Study the drawing (mm; zero at the part's minimum x, y, z) and answer. A direction names the side the tool comes from. Coordinates: 2 decimals unless noted, no trailing zeros. Write each loop counter-clockwise with the first axis right and the second up, starting at its lowest first coordinate (ties: lowest second). Pieces come first, ordered by that corner, then holes. Notation, with made-up numbers: (4.25, 42) -> (52.25, 42) arc R10 ccw to (52.25, 52) -> close; hole circle Ø9 at (-30, 33.25). An arc over 180 degrees is marked (long way). Write item = value, one per line. Start each with the question number.
1) Section B-B (x = 20) is taken. Determine the outline of the cut face in (y, z), plus the area to 3 significant figures.
2) Section C-C (y = 12) is taken. Determine the outline of the cut face in (x, z).
3) For a pull along Y with two mould halves and no side action, classify the marked faces 1, 2 and 3 as released by +Y, released by -Y, zero draft, split by the parting line, or undercut.
4) Section A-A (z = 17.25) is taken. Determine the outline of the cut face in (x, y), plus the area to 3 significant figures.
5) Section D-D (z = 3.75) is taken. Determine the outline of the cut face in (x, y).
6) Flat-ended cylindrical pins translate along their axes: pin 1 Ø6 at (y, z) = (35, 20.5) entering from -X; pin 2 Ø7.5 at (x, y) = (20, 19.5) entering from +Z; pin 3 Ø4 at (x, z) = (29, 16.5) entering from -Y (3 decimals). Find the tip coordinate at first contact, or state that the pin passes through.
7) Find the intervals of material crossed by line 1 along Z through (x, y) = (16, 12.5); line 2 along Y through (x, z) = (20, 14.5); line 3 along X through (y, z) = (23.5, 10.5), in increasing order. Write a range as from..to.
8) A tool of negligible diameter and unlimited length cuts with its end or side. For the marked faces 4 and 5, from which of +Z, -Z, +X, -X, +Y, -Y can it reach the whole face along a straight path? Write none if from no direction.
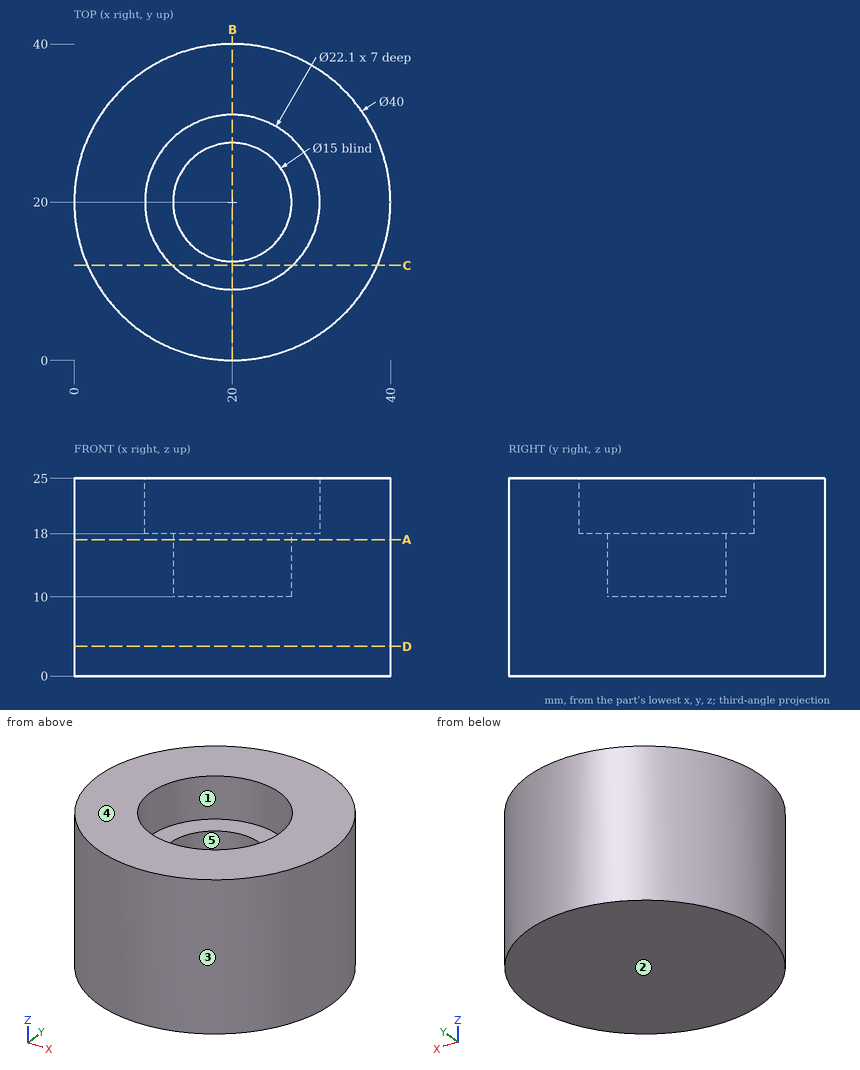
Answer key:
q1.outline = (0, 0) -> (40, 0) -> (40, 25) -> (31.05, 25) -> (31.05, 18) -> (27.5, 18) -> (27.5, 10) -> (12.5, 10) -> (12.5, 18) -> (8.95, 18) -> (8.95, 25) -> (0, 25) -> close
q1.area = 725 mm^2
q2.outline = (1.67, 0) -> (38.33, 0) -> (38.33, 25) -> (27.62, 25) -> (27.62, 18) -> (12.38, 18) -> (12.38, 25) -> (1.67, 25) -> close
q3.face_1 = undercut
q3.face_2 = zero draft
q3.face_3 = split by the parting line
q4.outline = circle Ø40 at (20, 20); hole circle Ø15 at (20, 20)
q4.area = 1,080 mm^2
q5.outline = circle Ø40 at (20, 20)
q6.pin_1 = 4
q6.pin_2 = 10
q6.pin_3 = 1.265
q7.line_1 = 0..18
q7.line_2 = 0..12.5, 27.5..40
q7.line_3 = 0.31..13.37, 26.63..39.69
q8.face_4 = +Z, +X, -X, +Y, -Y
q8.face_5 = +Z
